Part print with two shaded views. Sizes in mm from the minimum x, y, z corner. A direction names the side the tool comes from. Give positions to 0.01 mm unless a question says otherwise; leave off trailing zeros. Loops run counter-clockwise (first coordinate to the right, second up) from the corner with the lowest first, then second, coordinate; pieces in that order, holes last. Notation, with made-up numbers: M 36,50.5 L 65,50.5 A20 ccw 65,63.5 Z; hole C -22,39 d8. An arc over 180 degrees is marked long. Answer as a JSON object with one key per item and string values. Group by question number.
1. 3-axis set-ups, long thin cutter, end or side, ignore diameter. For the marked faces 1 and 2: which of +Z, -Z, +X, -X, +Y, -Y reach the whole face in a straight line?
2. Slice it at B-B (z = 4.75). List the corners of the cut face in (x, y), then the cut area to 3 significant figures.
3. Slice it at C-C (x = 26). List the corners of the cut face in (y, z).
4. Slice it at A-A (y = 8.75). List the corners of the cut face in (x, z), then the cut area to 3 significant figures.
5. Drill centre lines: line 1 along X through (y, z) = (4, 7.25); line 2 along Y through (x, z) = (21.5, 5.5). Where is each one in solid material? Low to high. Write a range as [from, to].
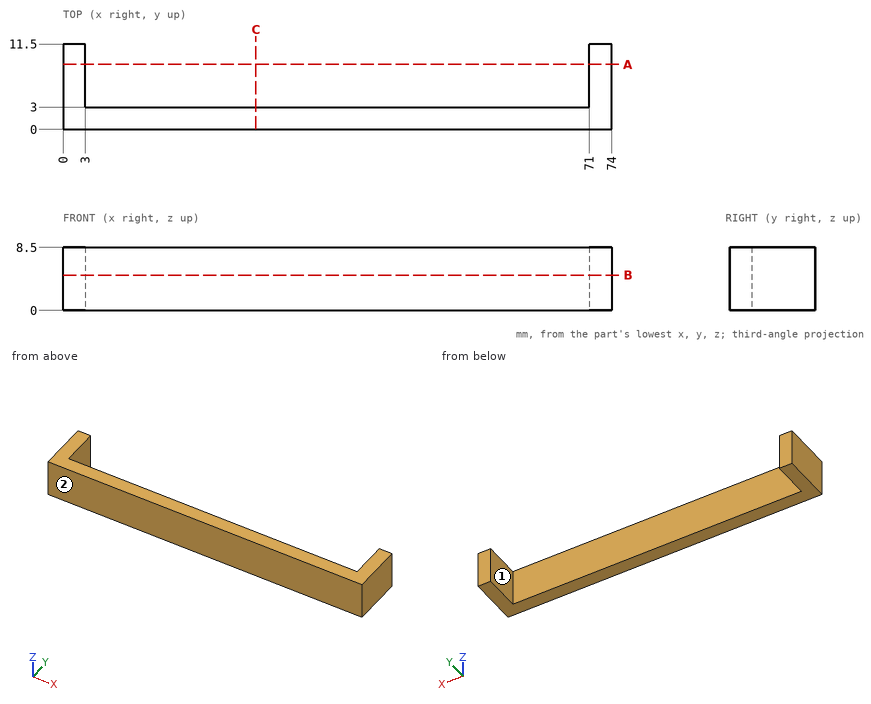
Established:
{
 "1": {"face 1": "+Z, -Z, +Y", "face 2": "+Z, -Z, +X, -X, -Y"},
 "2": {"outline": "M 0,0 L 74,0 L 74,11.5 L 71,11.5 L 71,3 L 3,3 L 3,11.5 L 0,11.5 Z", "area": "273 mm^2"},
 "3": {"outline": "M 0,0 L 3,0 L 3,8.5 L 0,8.5 Z"},
 "4": {"outline": "M 0,0 L 3,0 L 3,8.5 L 0,8.5 Z; M 71,0 L 74,0 L 74,8.5 L 71,8.5 Z", "area": "51.0 mm^2"},
 "5": {"line 1": "x = [0, 3], [71, 74]", "line 2": "y = [0, 3]"}
}
